Part model, mm, in its own coordinate system. A direction names the side the tool comes from. Coordinates: 2 decimals unless noted, no trailing zeros. Loops run counter-clockwise (first coordinate to the right, second up) from the corner with the lowest first, then second, coordinate; pieces in that order, holes last. Notation, with made-up numbers: (26.5, 15.5) - (32.5, 15.5) arc R12 ccw to (32.5, 35.5) - close; hole circle Ø5 at (5, -1.75). An arc over 180 degrees is marked (long way). Use a Markdown table: item, result. Add a question column.
1) Pull direction Y, two halves, no side cores. Call faces 4 (the face through (0, -3, 0)), 5 (the face through (7.4, -2.75, -18.5)), 6 (the face through (-8.3, -1.84, -23.21)): +Y half, -Y half, draft (parallel to the pull), parting line (faces both ways), or undercut.
2) Drop flat-ended pins along their axis: P1, Ø4, axis at y = 2.5, z = -18.5, coming from the -X side; P2, Ø6.5, axis at x = 0, y = 0, coming from the -Z side; P3, Ø1.3, axis at x = 7.5, z = -16, coming from the +Y side. Give the stop position or say it passes through.
3) Band-saw the part on B-B (y = -1). Give the number of separate pieces and of enclosed holes in the cut face, plus the area to 3 significant figures.
4) Band-saw the part on C-C (z = -19.5). Give the cut face in (x, y), plus the area to 3 significant figures.
5) Tool access for faces 1 (the face through (0, 3, -2)), 2 (the face through (7.672, -2.037, -25.848)), 3 (the face through (-2.685, -0.596, -0.986)): list every direction of +Z, -Z, +X, -X, +Y, -Y with a clear straight run to the whole face (end or side of a thin tool).
6) Band-saw the part on A-A (z = -30.5). Give the cut face in (x, y), plus the area to 3 significant figures.
7) Probe probe 1 along X at (y, z) = (0, -34); probe 2 along X at (y, z) = (0, -1.35). List the from-to ranges inside material, lowest first. Write a range as [from, to].
from build123d import *

# Parameters (mm, degrees)
CUT_EXTRUDE_1_DEPTH = 9.5
CHAMFER_1_SIZE      = 0.8


with BuildPart() as part:
    # Эскиз1 → Повернуть1 (revolve)
    with BuildSketch(Plane(origin=(0, 0, 0), x_dir=(0, 0, -1), z_dir=(1, 0, 0))):
        Polygon((0, 2.75), (0, 8.5), (45, 8.5), (45, 7.4), (2, 7.4), (2, 2.75), align=None)
    revolve(axis=Axis((0, 0, 0), (0, 0, -1)))

    # Эскиз2 → Вырез-Вытянуть1 (cut, through all)
    with BuildSketch(Plane(origin=(0, 0, 0), x_dir=(0, 0, -1), z_dir=(1, 0, 0))):
        with BuildLine():
            Line((13.1, -2.75), (24.1, -2.75))
            ThreePointArc((24.1, -2.75), (25.867766953, -2.017766953), (26.6, -0.25))
            Line((26.6, -0.25), (26.6, 0.25))
            ThreePointArc((26.6, 0.25), (25.867766953, 2.017766953), (24.1, 2.75))
            Line((24.1, 2.75), (13.1, 2.75))
            ThreePointArc((13.1, 2.75), (11.332233047, 2.017766953), (10.6, 0.25))
            Line((10.6, 0.25), (10.6, -0.25))
            ThreePointArc((10.6, -0.25), (11.332233047, -2.017766953), (13.1, -2.75))
        make_face()
    extrude(amount=CUT_EXTRUDE_1_DEPTH, mode=Mode.SUBTRACT)

    # Фаска1
    chamfer_1_edges = [part.edges().sort_by_distance(p)[0] for p in [
        (0, -8.5, 0),
    ]]
    chamfer(chamfer_1_edges, length=CHAMFER_1_SIZE)

    # Эскиз4 → Отверстие обработанное метчиком M2x0.41 (revolve, cut)
    with BuildSketch(Plane(origin=(-4.5, -4.5, 0), x_dir=(0, -1, 0), z_dir=(1, 0, 0))):
        Polygon((0, 0), (0, 2), (1.05, 2), (0.8, 1.75), (0.8, 0.3), (1.1, 0), align=None)
    revolve(axis=Axis((-4.5, -4.5, 6.35), (0, 0, -1)), mode=Mode.SUBTRACT)


solid = part.part
Answer block:
| question | item | result |
|---|---|---|
| 1 | face 4 | draft |
| 1 | face 5 | undercut |
| 1 | face 6 | parting line |
| 2 | P1 | x = -8.49 |
| 2 | P2 | z = -2 |
| 2 | P3 | y = 5.03 |
| 3 | separate pieces | 3 |
| 3 | enclosed holes | 0 |
| 3 | area | 101 mm2 |
| 4 | outline | (6.87, -2.75) arc R7.4 cw (long way) to (6.87, 2.75) - (8.04, 2.75) arc R8.5 ccw (long way) to (8.04, -2.75) - close |
| 4 | area | 48.8 mm2 |
| 5 | face 1 | -Z |
| 5 | face 2 | +X |
| 5 | face 3 | +Z, -Z |
| 6 | outline | circle Ø17 at (0, 0); hole circle Ø14.8 at (0, 0) |
| 6 | area | 54.9 mm2 |
| 7 | probe 1 | [-8.5, -7.4], [7.4, 8.5] |
| 7 | probe 2 | [-8.5, -2.75], [2.75, 8.5] |
